Autodesk Inventor part; units mm, degrees
ref_plane "YZ Plane" through (0, 0, 0) normal (1, 0, 0) x (0, 1, 0)
ref_plane "XZ Plane" through (0, 0, 0) normal (0, 1, 0) x (-1, 0, 0)
ref_plane "XY Plane" through (0, 0, 0) normal (0, 0, 1) x (1, 0, 0)
sketch "Sketch1" plane through (0, 0, 0) normal (0, 0, 1) x (1, 0, 0)
  line L0 (0, 0) -> (14, 0)
  line L1 (14, 0) -> (14, -14)
  line L2 (14, -14) -> (0, -14)
  line L3 (0, -14) -> (0, 0)
  dimension "d0" = 14
  dimension "d1" = 14
extrude "Extrusion1" add sketch "Sketch1" against normal blind 22
sketch "Sketch2" plane through (0, 0, 0) normal (0, 0, 1) x (1, 0, 0)
  line L0 (2, -2) -> (12, -2)
  line L1 (12, -2) -> (12, -22)
  line L2 (12, -22) -> (2, -22)
  line L3 (2, -22) -> (2, -2)
  point P0 (0, 0)
  dimension "d4" = 10
  dimension "d5" = 20
extrude "Extrusion2" cut sketch "Sketch2" against normal blind 20
sketch "Sketch8" plane through (0, -14, 0) normal (-1, 0, 0) x (0, 0, 1)
  point P0 (0, 14)
sketch "Sketch9" plane through (0, -14, 0) normal (-1, 0, 0) x (0, 0, 1)
  point P0 (0, 14)
sketch "Sketch11" plane through (0, -14, 0) normal (-1, 0, 0) x (0, 0, 1)
  point P0 (0, 14)
sketch "Sketch14" plane through (0, -14, 0) normal (-1, 0, 0) x (0, 0, 1)
  point P0 (0, 14)
sketch "Sketch15" plane through (0, -14, 0) normal (-1, 0, 0) x (0, 0, 1)
  point P0 (0, 14)
sketch "Sketch16" plane through (0, -14, 0) normal (-1, 0, 0) x (0, 0, 1)
  line L0 (-12.5, 12) -> (-17.5, 12)
  line L1 (-17.5, 12) -> (-17.5, 0)
  line L2 (-17.5, 0) -> (-12.5, 0)
  line L3 (-12.5, 0) -> (-12.5, 12)
  point P0 (0, 14)
  dimension "d30" = 5
  dimension "d31" = 12
extrude "Extrusion10" cut sketch "Sketch16" against normal blind 2
sketch "Sketch17" plane through (0, 0, -20) normal (0, 0, 1) x (1, 0, 0)
  line L0 (12, -2) -> (7.5, -2)
  line L1 (7.5, -2) -> (7.5, -6.5)
  line L2 (7.5, -6.5) -> (12, -6.5)
  line L3 (12, -6.5) -> (12, -2)
  point P0 (0, 0)
  dimension "d34" = 4.5
  dimension "d35" = 4.5
extrude "Extrusion11" add sketch "Sketch17" along normal blind 9
properties part number "housing_v06"
Source: CAD feature listing. Evaluate the final solid. Frame: model axes, mm. A direction names the side the tool comes from. Round coordinates to 2 decimals unless told otherwise and drop trailing zeros. Order: outer loops, then holes, each group sorted by start corner. A loop starts at its lowest first (then second) coordinate and runs counter-clockwise, first axis right, second up. Notation, with made-up numbers: (71.5, 56) -> (114.5, 56) arc R25 ccw to (114.5, 75) -> close; hole circle Ø3 at (13, 16.25). An arc over 180 degrees is marked (long way). One line per item, written item: value. Start each with the question number.
Q1. Pin query (flat end, axial travel): pin 1 (2 mm diameter, centred on x = 4, z = -6.5, fed in from -Y); pin 2 (2 mm diameter, centred on x = 9.5, y = -3.5, fed in from +Z); pin 3 (1 mm diameter, centred on x = 5.5, y = -10, fed in from +Z). Return the tip coordinate at first contact, or that it passes through.
Q2. Draft query along X for faces 1 (the flat face through (14, -7, -11)), 2 (the flat face through (12.2, -14, -14.2)), 3 (the flat face through (12, -9, -10)). Return one class per face: pulls with the +X half, pulls with the -X half, needs draft (parallel to the pull), parting line crosses it, or undercut.
Q3. Section query B-B (z = -3.75). Return the cut outline in (x, y), plus the area to 3 significant figures.
Q4. Section query C-C (x = 4.25). Return the cut outline in (y, z), plus the area to 3 significant figures.
Q5. Material intervals for probe 1 along X at (y, z) = (-8.25, -11.75); probe 2 along Z at (x, y) = (1.75, -13.5); probe 3 along Y at (x, z) = (7, -1.5), sorted ascending.
Q6. Access query for faces 4 (the flat face through (1, -8, -17.5)), 5 (the flat face through (1, -14, -6)), 6 (the flat face through (7.5, -4, -16)). Directions: +Z, -Z, +X, -X, +Y, -Y. A direction counts if a zero-diameter tool reaches every point of the face in a straight line with its end or side. Return the directions, or none.
Q7. Section query D-D (y = -11.75). Return the cut outline in (x, z), plus the area to 3 significant figures.
Q8. Section query A-A (y = -3.5). Return the cut outline in (x, z).
Findings below:
1. pin 1: y = -2
1. pin 2: z = -11
1. pin 3: z = -20
2. face 1: pulls with the +X half
2. face 2: needs draft
2. face 3: undercut
3. outline: (0, -14) -> (2, -14) -> (2, -2) -> (12, -2) -> (12, -14) -> (14, -14) -> (14, 0) -> (0, 0) -> close
3. area: 76.0 mm²
4. outline: (-14, -22) -> (0, -22) -> (0, 0) -> (-2, 0) -> (-2, -20) -> (-14, -20) -> close
4. area: 68.0 mm²
5. probe 1: 0 to 2, 12 to 14
5. probe 2: -22 to -17.5, -12.5 to 0
5. probe 3: -2 to 0
6. face 4: -X, -Y
6. face 5: +Z, -Z, +X, -X, -Y
6. face 6: +Z, -Y
7. outline: (0, -22) -> (14, -22) -> (14, 0) -> (12, 0) -> (12, -20) -> (2, -20) -> (2, -17.5) -> (0, -17.5) -> close; (0, -12.5) -> (2, -12.5) -> (2, 0) -> (0, 0) -> close
7. area: 98.0 mm²
8. outline: (0, -22) -> (14, -22) -> (14, 0) -> (12, 0) -> (12, -11) -> (7.5, -11) -> (7.5, -20) -> (2, -20) -> (2, -17.5) -> (0, -17.5) -> close; (0, -12.5) -> (2, -12.5) -> (2, 0) -> (0, 0) -> close
